Autodesk Inventor part; units mm, degrees
ref_plane "YZ Plane" through (0, 0, 0) normal (1, 0, 0) x (0, 1, 0)
ref_plane "XZ Plane" through (0, 0, 0) normal (0, 1, 0) x (-1, 0, 0)
ref_plane "XY Plane" through (0, 0, 0) normal (0, 0, 1) x (1, 0, 0)
sketch "Sketch1" plane through (0, 0, 0) normal (0, 0, 1) x (1, 0, 0)
  line L0 (-15, 18.5) -> (15, 18.5)
  line L1 (-15, 18.5) -> (-15, 0)
  line L2 (15, 18.5) -> (15, 0)
  line L3 (-30, 0) -> (-15, 0)
  line L4 (15, 0) -> (30, 0)
  point P0 (0, 0)
  dimension "d0" = 30
  dimension "d1" = 15
  dimension "d3" = 18.5
  dimension "d4" = 15
  dimension "d5" = 15
contour flange "Contour Flange1" sketch "Sketch1" thickness 1.5 bend radius 1.5 width 245 along (0, 0, 1) mid plane yes both sides no wall seen from (-22.5, 0, 0) lies toward (0, 1, 0) curves L3 L1 L0 L2 L4
bend "Bend1"
corner "Corner1"
equation "\"d6\" = BendReliefWidth"
equation "\"d7\" = BendReliefDepth"
equation "\"d8\" = MinimumRemnant"
equation "\"d9\" = BendRadius"
equation "\"d11\" = BendRadius"
equation "\"d13\" = CornerReliefSize"
equation "\"d14\" = GapSize"
equation "\"d15\" = JacobiRadiusSize"
equation "\"BendRadius\" = Thickness"
equation "\"BendReliefWidth\" = Thickness"
equation "\"BendReliefDepth\" = 0.5 * Thickness"
equation "\"CornerReliefSize\" = 4 * Thickness"
equation "\"MinimumRemnant\" = 2 * Thickness"
equation "\"TransitionRadius\" = BendRadius"
equation "\"JacobiRadiusSize\" = BendRadius"
equation "\"GapSize\" = Thickness"
properties part number "Reforço Bandeja" material "Stainless Steel AISI 304"
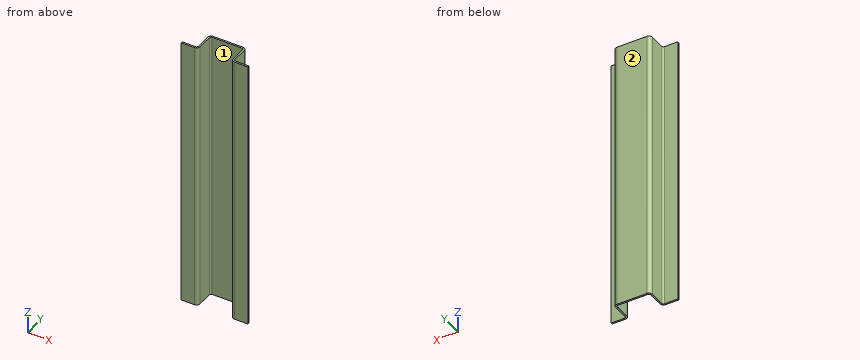
Geometry check sheet. Reference: the model listing, model coordinates, mm. Face numbers are marked on the shaded views. Round coordinates to 2 decimals unless told otherwise and drop trailing zeros. Order: outer loops, then holes, each group sorted by start corner. A loop starts at its lowest first (then second) coordinate and runs counter-clockwise, first axis right, second up. Notation, with made-up numbers: M 60,51 L 93,51 A27 ccw 93,89 Z; hole C 55,64.5 d5. An arc over 180 degrees is marked long. Answer in a Markdown table with one row per item. Add a question column.
Item 1: Draft check along X on the marked faces 1 and 2. Enter one of: released by +X, released by -X, zero draft, split by the parting line, or undercut.
Item 2: Sectioned sample at B-B, the plane z = -67. Enter the section's corners in (x, y).
Item 3: Sectioned sample at A-A, the plane y = 13.75. Enter the section's corners in (x, z), plus the area to 3 significant figures.
Item 4: Depth check by flat-ended pin: pin 1 Ø4 at (y, z) = (13.5, 47) entering from -X; pin 2 Ø2 at (y, z) = (11.5, 73) entering from +X; pin 3 Ø13 at (x, z) = (24.5, -54.5) entering from +Y. Enter the tip coordinate at first touch or a pass-through.
Item 5: Material ranges on L1, parallel to X at y = 11.5, z = 61; L2, parallel to Y at x = -13.5, z = -110.5; L3, parallel to Y at x = 21.5, z = -53, recorded low to high. Write a range as [from, to].
Item 6: Sectioned sample at C-C, the plane x = 5. Enter the section's corners in (y, z), plus the area to 4 significant figures.
Filled in:
| question | item | result |
|---|---|---|
| 1 | face 1 | undercut |
| 1 | face 2 | zero draft |
| 2 | outline | M -30,0 L -18,0 A3 ccw -15,3 L -15,17 A1.5 cw -13.5,18.5 L 13.5,18.5 A1.5 cw 15,17 L 15,3 A3 ccw 18,0 L 30,0 L 30,1.5 L 18,1.5 A1.5 cw 16.5,3 L 16.5,17 A3 ccw 13.5,20 L -13.5,20 A3 ccw -16.5,17 L -16.5,3 A1.5 cw -18,1.5 L -30,1.5 Z |
| 3 | outline | M -16.5,-122.5 L -15,-122.5 L -15,122.5 L -16.5,122.5 Z; M 15,-122.5 L 16.5,-122.5 L 16.5,122.5 L 15,122.5 Z |
| 3 | area | 735 mm² |
| 4 | pin 1 | stops at x = -16.5 |
| 4 | pin 2 | stops at x = 16.5 |
| 4 | pin 3 | stops at y = 1.5 |
| 5 | L1 | x = [-16.5, -15], [15, 16.5] |
| 5 | L2 | y = [18.5, 20] |
| 5 | L3 | y = [0, 1.5] |
| 6 | outline | M 18.5,-122.5 L 20,-122.5 L 20,122.5 L 18.5,122.5 Z |
| 6 | area | 367.5 mm² |
